Autodesk Inventor part; units mm, degrees
ref_plane "WorkPlane8" through (0, 0, 0) normal (1, 0, 0) x (0, 1, 0)
ref_plane "WorkPlane7" through (0, 0, 0) normal (0, 1, 0) x (-1, 0, 0)
ref_plane "XY Plane" through (0, 0, 0) normal (0, 0, 1) x (1, 0, 0)
sketch "Sketch2" plane through (0, 0, 0) normal (0, 0, 1) x (1, 0, 0)
  circle A0 centre (0, 0) radius 4
  dimension "d1" = 8
extrude "Extrusion1" add sketch "Sketch2" against normal blind 17
chamfer "Chamfer1" distance 1.6 angle 15 1 edges at (-4, 0, -17) measured on face at (3.9482, -0.6416, -11.3333)
sketch "Sketch3" plane through (0, 0, 0) normal (0, 0, 1) x (1, 0, 0)
  circle A0 centre (0, 0) radius 4
  circle A1 centre (0, 0) radius 4 construction
  dimension "d7" = 8
extrude "Extrusion2" add sketch "Sketch3" along normal blind 1 draft -15
sketch "Sketch4" plane through (0, 0, 1) normal (0, 0, 1) x (1, 0, 0)
  circle A0 centre (0, 0) radius 2.65
  circle A1 centre (0, 0) radius 3.7321 construction
  dimension "d13" = 5.3
extrude "Extrusion3" cut sketch "Sketch4" against normal blind 1.2
sketch "Sketch5" plane through (0, 0, -0.2) normal (0, 0, 1) x (1, 0, 0)
  circle A0 centre (0, 0) radius 2.65
hole "Hole1" at (0, 0, -0.2) direction (0, 0, -1) diameter 4.134 depth 10.7134 tip angle 118 countersink diameter 5.3 countersink angle 120
equation "\"d4\" = c2"
equation "\"d30\" = c2"
equation "\"d2\" = -c1 + NLG"
equation "\"d7\" = Diam1"
equation "\"d8\" = c1"
equation "\"d13\" = Diam3"
equation "\"d14\" = t3"
equation "\"d19\" = -t3 + t1 + 0.288675 * Diam2 - 0.288675 * Diam3"
equation "\"d20\" = Diam3"
equation "\"d23\" = -t3 + t2 + 0.288675 * Diam2 - 0.288675 * Diam3"
equation "\"d1\" = Diam1"
equation "\"Diam1\" = 8"
equation "\"Diam2\" = 5"
equation "\"Diam3\" = 5.3"
equation "\"t1\" = 8"
equation "\"t2\" = 12"
equation "\"t3\" = 1.2"
equation "\"NLG\" = 18"
equation "\"c1\" = 1"
equation "\"c2\" = 1.6"
equation "\"P\" = 1"
equation "\"THREADDIA\" = Diam2"
equation "\"PTC\" = 0.8"
properties part number "CSN EN ISO 8733 - 8x18-St" material "Stainless Steel, Austenitic"
Here's how the part is built. I have some questions about the finished solid (model axes, mm). A direction names the side the tool comes from. Round coordinates to 2 decimals unless told otherwise and drop trailing zeros. Write each loop counter-clockwise with the first axis right and the second up, starting at its lowest first coordinate (ties: lowest second). Pieces come first, ordered by that corner, then holes.
1. Suppose I cut it at A-A (z = -13.5). List the corners of the cut face in (x, y) for me, and give its area (3 significant figures).
2. I need wall thicknesses on L1, parallel to Y at x = 0, z = -3; L2, parallel to X at y = 0, z = 0.45; L3, parallel to X at y = 0.25, z = -4.75. Which ranges of each line are inside material? Lowest first, please.
3. Suppose I cut it at B-B (z = -4). List the corners of the cut face in (x, y) for me.
4. Will these pins go through, and if not, where does the flat tip stop? pin 1 Ø1 at (x, z) = (-3, -9.5) entering from +Y; pin 2 Ø3 at (x, z) = (2.5, -11) entering from +Y.
5. If we mould it in two halves opening along X, with no side actions, what happens to faces 3 (the flat face through (1, 3, 1)), 4 (the cylindrical face through (-0.867, -3.905, -7.592)), 5 (the cylindrical face through (2.45, -1.01, 0.41))? For each: released by +X, released by -X, zero draft, split by the parting line, or undercut.
6. For faces 1 (the cylindrical face through (1.26, 1.64, -5.8)), 2 (the flat face through (0, 0, -17)), which set-ups out of +Z, -Z, +X, -X, +Y, -Y let a thin tool reach every point of the face, with its end or its side?
Answer sheet:
1. outline: circle Ø8 at (0, 0)
1. area: 50.3 mm2
2. L1: y = -4 to -2.07, 2.07 to 4
2. L2: x = -3.88 to -2.65, 2.65 to 3.88
2. L3: x = -3.99 to -2.05, 2.05 to 3.99
3. outline: circle Ø8 at (0, 0); hole circle Ø4.13 at (0, 0)
4. pin 1: stops at y = 3.12
4. pin 2: stops at y = 3.87
5. face 3: zero draft
5. face 4: split by the parting line
5. face 5: undercut
6. face 1: +Z
6. face 2: -Z, +X, -X, +Y, -Y
